The listing builds one solid part. Answer for the finished solid, in the listing's coordinates (mm). Coordinates: 2 decimals unless noted, no trailing zeros. Order: outer loops, then holes, each group sorted by start corner. A loop starts at its lowest first (then second) coordinate and runs counter-clockwise, first axis right, second up. Notation, with made-up numbers: (-9, -26) -> (-4, -26) arc R20 ccw to (-4, 9) -> close; hole circle Ø2 at (40, 50). An arc over 180 degrees is marked (long way). Write item = value, one per line.
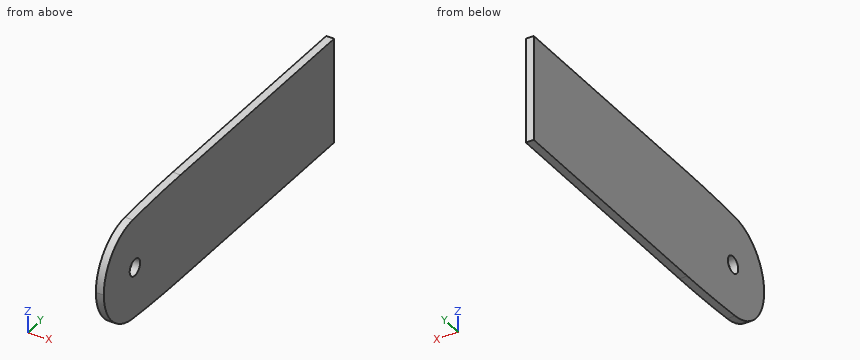
Autodesk Inventor part; units mm, degrees
ref_plane "YZ Plane" through (0, 0, 0) normal (1, 0, 0) x (0, 1, 0)
ref_plane "XZ Plane" through (0, 0, 0) normal (0, 1, 0) x (-1, 0, 0)
ref_plane "XY Plane" through (0, 0, 0) normal (0, 0, 1) x (1, 0, 0)
sketch "Sketch1" plane through (0, 0, 0) normal (1, 0, 0) x (0, 1, 0)
  line L0 (122, 20) -> (28, 20)
  arc A0 (28, 20) -> (-1.2912, 19.0062) centre (28, -412.1566) ccw
  arc A1 (-1.2912, 19.0062) -> (-19.05, 0) centre (0, 0) ccw
  line L1 (-19.05, 0) -> (122, 0)
  line L2 (122, 0) -> (122, 20)
  circle A2 centre (0, 0) radius 3.175
  point P0 (-3.175, 0)
  point P1 (3.175, 0)
  dimension "d0" = 19.05
  dimension "d1" = 6.35
  dimension "d2" = 122
  dimension "d3" = 94
  dimension "d4" = 20
extrude "Extrusion1" add sketch "Sketch1" along normal blind 3 contours L2 L1 A2 A1 A0 L0
mirror "Mirror1" about plane through (0, 0, 0) normal (0, 0, 1) of "Extrusion1"
properties part number "wristPlate"
Q1. Section B-B, the plane y = 0 is taken. Give the vertices of the cut face in (x, z) (3 decimals).
The answers:
outline = (0, -19.092) -> (3, -19.092) -> (3, -3.175) -> (0, -3.175) -> close; (0, 3.175) -> (3, 3.175) -> (3, 19.092) -> (0, 19.092) -> close
Q2. Find the intervals of material crossed by line 1 along Y through (x, z) = (2.45, 0) (3 decimals); line 2 along Z through (x, y) = (1.1, 25); line 3 along Z through (x, y) = (2.45, 0) (3 decimals), in increasing order.
The answers:
line_1 = -19.05 to -3.175, 3.175 to 122
line_2 = -19.99 to 19.99
line_3 = -19.092 to -3.175, 3.175 to 19.092
Q3. Section A-A, the plane x = 1.85 is taken. Give the vertices of the cut face in (y, z) (3 decimals).
The answers:
outline = (-19.05, 0) arc R19.05 ccw to (-1.291, -19.006) arc R432.164 ccw to (28, -20) -> (122, -20) -> (122, 20) -> (28, 20) arc R432.164 ccw to (-1.291, 19.006) arc R19.05 ccw to start; hole circle Ø6.35 at (0, 0)
Q4. Section C-C, the plane z = 11.5 is taken. Give the vertices of the cut face in (x, y).
The answers:
outline = (0, -15.19) -> (3, -15.19) -> (3, 122) -> (0, 122) -> close
Q5. Section D-D, the plane z = -16 is taken. Give the vertices of the cut face in (x, y), plus the area to 3 significant figures.
The answers:
outline = (0, -10.34) -> (3, -10.34) -> (3, 122) -> (0, 122) -> close
area = 397 mm2
